Source: CAD feature listing. Evaluate the final solid. Frame: model axes, mm. A direction names the side the tool comes from. Coordinates: 2 decimals unless noted, no trailing zeros. Loops run counter-clockwise (first coordinate to the right, second up) from the corner with the lowest first, then second, coordinate; pieces in that order, holes last. Notation, with made-up numbers: (15, 25) -> (51, 25) arc R34 cw to (51, 62) -> close; hole circle Ø4 at (2.25, 59). An arc over 180 degrees is marked (long way). Answer as a JSON object with one key per item and string values. Group by question number.
from build123d import *

# Parameters (mm, degrees)
SKETCH1_R             = 1.5
BOSS_EXTRUDE3_DEPTH   = 8
BOSS_EXTRUDE3_2_DEPTH = 8
SKETCH4_W             = 35
SKETCH4_H             = 20
BOSS_EXTRUDE4_DEPTH   = 16


with BuildPart() as part:
    # Sketch1 → Boss-Extrude3 (new body)
    with BuildSketch(Plane(origin=(0, 0, 0), x_dir=(1, 0, 0), z_dir=(0, 1, 0))):
        Polygon((32.5, -10), (32.5, 10), (17.5, 10), (17.5, 5), (17.5, -5), (17.5, -10), align=None)
        with BuildLine():
            ThreePointArc((24, -5), (22.5, -6.5), (21, -5))
            ThreePointArc((21, -5), (22.5, -3.5), (24, -5))
        make_face(mode=Mode.SUBTRACT)
        with Locations((29.5, -5)):
            Circle(SKETCH1_R, mode=Mode.SUBTRACT)
        with BuildLine():
            ThreePointArc((24, 5), (22.5, 3.5), (21, 5))
            ThreePointArc((21, 5), (22.5, 6.5), (24, 5))
        make_face(mode=Mode.SUBTRACT)
        with Locations((29.5, 5)):
            Circle(SKETCH1_R, mode=Mode.SUBTRACT)
    extrude(amount=BOSS_EXTRUDE3_DEPTH)



with BuildPart() as body_2:
    # Sketch1 → Boss-Extrude3 2 (new body)
    with BuildSketch(Plane(origin=(0, 0, 0), x_dir=(1, 0, 0), z_dir=(0, 1, 0))):
        Polygon((-17.5, 5), (-17.5, 10), (-32.5, 10), (-32.5, -10), (-17.5, -10), align=None)
        with BuildLine():
            ThreePointArc((-28, -5), (-30.560660172, -6.060660172), (-29.5, -3.5))
            ThreePointArc((-29.5, -3.5), (-28.439339828, -3.939339828), (-28, -5))
        make_face(mode=Mode.SUBTRACT)
        with Locations((-22.5, -5)):
            Circle(SKETCH1_R, mode=Mode.SUBTRACT)
        with BuildLine():
            ThreePointArc((-29.5, 3.5), (-30.560660172, 6.060660172), (-28, 5))
            ThreePointArc((-28, 5), (-28.439339828, 3.939339828), (-29.5, 3.5))
        make_face(mode=Mode.SUBTRACT)
        with BuildLine():
            ThreePointArc((-24, 5), (-22.5, 6.5), (-21, 5))
            ThreePointArc((-21, 5), (-22.5, 3.5), (-24, 5))
        make_face(mode=Mode.SUBTRACT)
    extrude(amount=BOSS_EXTRUDE3_2_DEPTH)


with BuildPart() as part_1:
    add(part.part)

    add(body_2.part)  # Boss-Extrude4 merges body 2
    # Sketch4 → Boss-Extrude4 (add)
    with BuildSketch(Plane.XZ):
        Rectangle(SKETCH4_W, SKETCH4_H)
    extrude(amount=-BOSS_EXTRUDE4_DEPTH)


solid = part_1.part
1. Ray query, L1, parallel to Z at x = 29.5, y = 3.5; L2, parallel to X at y = 1.5, z = 5; L3, parallel to X at y = 7.5, z = -3.75. Return the intervals inside material, ascending.
2. Section query A-A on x = 29.5. Return loops of the section in (y, z).
3. Section query B-B on y = 5.5. State how many separate pieces and enclosed holes the cut face has, then the cut area to 3 significant figures.
4. Section query C-C on z = -8.5. Return loops of the section in (x, y), then the cut area to 3 significant figures.
5. Reachability of faces 1 (the face through (32.5, 4, 0)), 2 (the face through (-17.5, 12, 0)), 3 (the face through (25, 8, 0)) from +Z, -Z, +X, -X, +Y, -Y: full face, straight path, thin tool, end or side. Return the list, or none.
6. Section query D-D on x = -26. Return loops of the section in (y, z).
7. Pin query (flat end, axial travel): pin 1 Ø4 at (x, z) = (-22.5, 5) entering from +Y; pin 2 Ø2.5 at (x, z) = (-29.5, -5) entering from -Y; pin 3 Ø2.5 at (y, z) = (13, 2) entering from -X. Return the tip coordinate at first contact, or that it passes through.
8. Mould query, pull axis Z, two halves, no side actions, for faces 4 (the face through (17.5, 12, 0)), 5 (the face through (0, 6, 10)), 6 (the face through (28, 4, -5)), 7 (the face through (24, 4, -5)). Classes: pulls with the +Z half, pulls with the -Z half, needs draft (parallel to the pull), parting line crosses it, or undercut.
Solved:
{
 "1": {"L1": "-10 to -6.5, -3.5 to 3.5, 6.5 to 10", "L2": "-32.5 to -31, -28 to -24, -21 to 21, 24 to 28, 31 to 32.5", "L3": "-32.5 to -30.33, -28.67 to -23.33, -21.67 to 21.67, 23.33 to 28.67, 30.33 to 32.5"},
 "2": {"outline": "(0, -10) -> (8, -10) -> (8, -6.5) -> (0, -6.5) -> close; (0, -3.5) -> (8, -3.5) -> (8, 3.5) -> (0, 3.5) -> close; (0, 6.5) -> (8, 6.5) -> (8, 10) -> (0, 10) -> close"},
 "3": {"separate pieces": "1", "enclosed holes": "8", "area": "1,240 mm^2"},
 "4": {"outline": "(-32.5, 0) -> (32.5, 0) -> (32.5, 8) -> (17.5, 8) -> (17.5, 16) -> (-17.5, 16) -> (-17.5, 8) -> (-32.5, 8) -> close", "area": "800 mm^2"},
 "5": {"face 1": "+Z, -Z, +X, +Y, -Y", "face 2": "+Z, -Z, -X, +Y", "face 3": "+Z, -Z, +X, +Y"},
 "6": {"outline": "(0, -10) -> (8, -10) -> (8, 10) -> (0, 10) -> close"},
 "7": {"pin 1": "y = 8", "pin 2": "through", "pin 3": "x = -17.5"},
 "8": {"face 4": "needs draft", "face 5": "pulls with the +Z half", "face 6": "undercut", "face 7": "undercut"}
}
